Check sheet for the drawn part. Datum: minimum x, y, z corner. Units: mm. Round coordinates to 2 decimals unless told otherwise and drop trailing zeros. Order: outer loops, then holes, each group sorted by start corner. A loop starts at its lowest first (then second) coordinate and runs counter-clockwise, first axis right, second up.
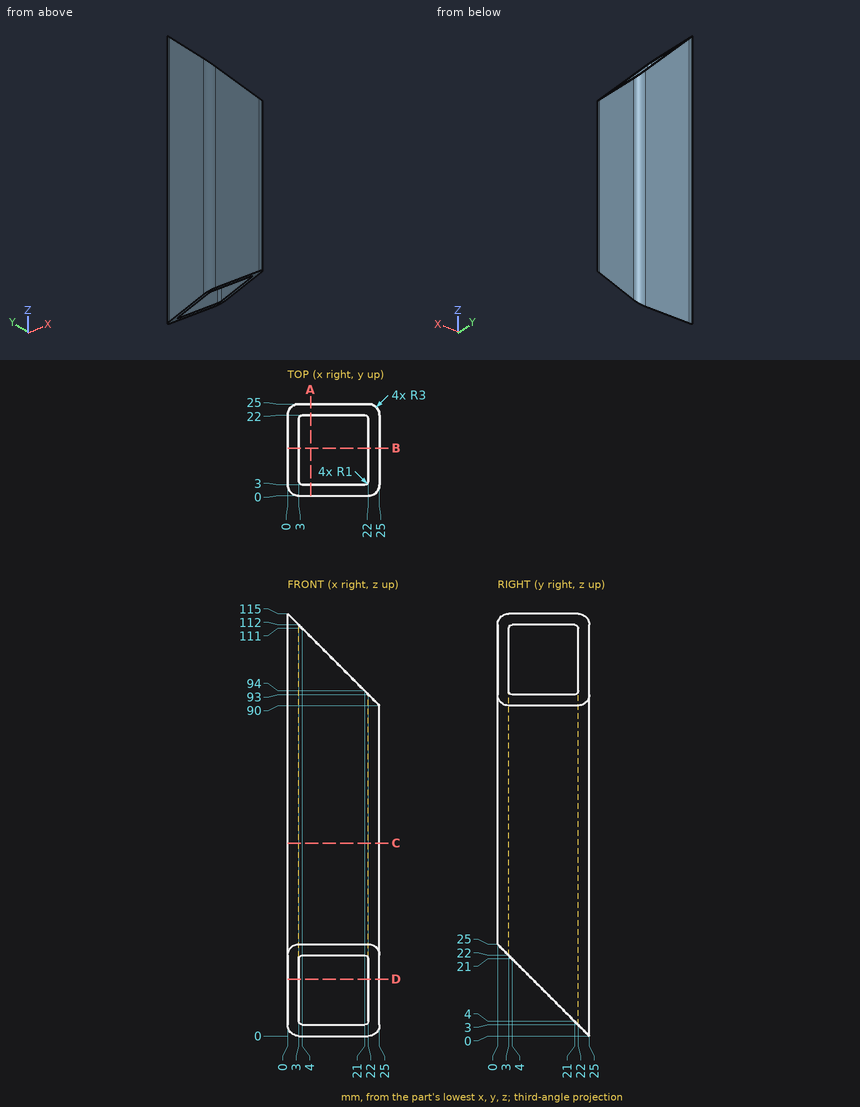
1) Sectioned sample at C-C on z = 52.5. Record the cut outline in (x, y), and give its area (3 significant figures).
2) Sectioned sample at D-D on z = 15.5. Record the cut outline in (x, y), and give its area (3 significant figures).
3) Sectioned sample at A-A on x = 6.25. Record the cut outline in (y, z), and give its area (4 significant figures).
4) Scan lines: line 1 (Y direction, x = 9.25, z = 64); line 2 (Y direction, x = 17, z = 7.5). Record each from-to range of solid material in increasing order.
5) Sectioned sample at B-B on y = 13. Record the cut outline in (x, z).
6) Gauge pin test, flat end, axial feed: pin 1 (6 mm diameter, centred on x = 19.5, y = 15, fed in from +Z). Record the tip position at first contact, or that the pin passes through.
Values found:
1. outline: (0, 3) arc R3 ccw to (3, 0) - (22, 0) arc R3 ccw to (25, 3) - (25, 22) arc R3 ccw to (22, 25) - (3, 25) arc R3 ccw to (0, 22) - close; hole (3, 4) arc R1 ccw to (4, 3) - (21, 3) arc R1 ccw to (22, 4) - (22, 21) arc R1 ccw to (21, 22) - (4, 22) arc R1 ccw to (3, 21) - close
1. area: 257 mm2
2. outline: (0, 9.5) - (3, 9.5) - (3, 21) arc R1 cw to (4, 22) - (21, 22) arc R1 cw to (22, 21) - (22, 9.5) - (25, 9.5) - (25, 22) arc R3 ccw to (22, 25) - (3, 25) arc R3 ccw to (0, 22) - close
2. area: 147 mm2
3. outline: (0, 25) - (3, 22) - (3, 108.75) - (0, 108.75) - close; (22, 3) - (25, 0) - (25, 108.75) - (22, 108.75) - close
3. area: 577.5 mm2
4. line 1: y = 0 to 3, 22 to 25
4. line 2: y = 22 to 25
5. outline: (0, 12) - (3, 12) - (3, 112) - (0, 115) - close; (22, 12) - (25, 12) - (25, 90) - (22, 93) - close
6. pin 1: stops at z = 93
